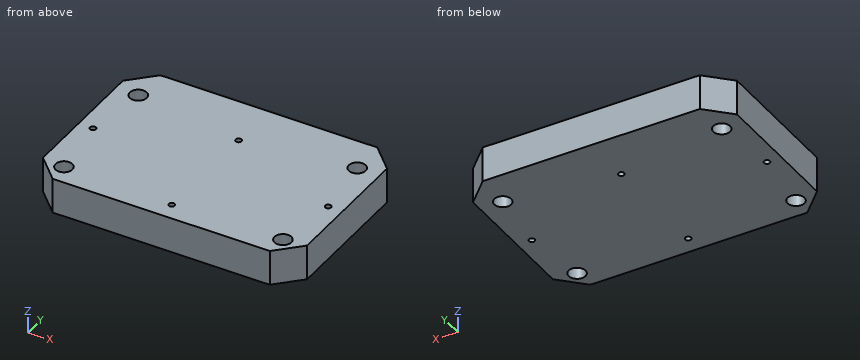
from build123d import *

# Parameters (mm, degrees)
SKETCH1_W                        = 142.628975504
SKETCH1_H                        = 98.843650928
BOSS_EXTRUDE1_DEPTH              = 19.05
CHAMFER1_SIZE                    = 12.7
F_23_64_0_35938_DIAMETER_HOLE1_D = 9.128252
HOLE1_D                          = 3.175
HOLE1_DEPTH                      = 44.45
HOLE1_CSINK_D                    = 10.16
HOLE1_CSINK_ANGLE                = 82
HOLE1_TIP                        = 0.953866233


with BuildPart() as part:
    # Sketch1 → Boss-Extrude1 (new body)
    with BuildSketch(Plane.XY):
        with Locations((0, 439.814227158)):
            Rectangle(SKETCH1_W, SKETCH1_H)
    extrude(amount=BOSS_EXTRUDE1_DEPTH)

    # Chamfer1
    chamfer1_edges = [part.edges().sort_by_distance(p)[0] for p in [
        (71.314487752, 390.392401694, 9.525),
        (-71.314487752, 390.392401694, 9.525),
        (-71.314487752, 489.236052622, 9.525),
        (71.314487752, 489.236052622, 9.525),
    ]]
    chamfer(chamfer1_edges, length=CHAMFER1_SIZE)

    # 23/64 (0.35938) Diameter Hole1 (through all)
    with Locations(Plane.XY.offset(19.05)):
        with Locations((-59.12, 469.942526688), (59.12, 469.942526688), (59.12, 401.616526688), (-59.12, 401.616526688)):
            Hole(F_23_64_0_35938_DIAMETER_HOLE1_D / 2)

    # Hole1
    with Locations(Plane(origin=(0, 0, -19.05), x_dir=(-1, 0, 0), z_dir=(0, 0, -1))):
        with Locations((63.5, 435.779526688), (-63.5, 435.779526688), (0, 461.558384256), (0, 400.075074406)):
            CounterSinkHole(HOLE1_D / 2, HOLE1_CSINK_D / 2, depth=HOLE1_DEPTH, counter_sink_angle=HOLE1_CSINK_ANGLE)
            with Locations((0, 0, -(HOLE1_DEPTH + HOLE1_TIP / 2))):  # 118° drill point
                Cone(0, HOLE1_D / 2, HOLE1_TIP, mode=Mode.SUBTRACT)


solid = part.part
Geometry: final body of the model. Coordinates: model frame, mm. Give positions to 0.01 mm unless a question says otherwise; leave off trailing zeros. Write each loop counter-clockwise with the first axis right and the second up, starting at its lowest first coordinate (ties: lowest second). Pieces come first, ordered by that corner, then holes. Notation, with made-up numbers: (70, 68.25) -> (125, 68.25) arc R16 ccw to (125, 87.25) -> close; hole circle Ø4 at (53.25, 46). An arc over 180 degrees is marked (long way). Answer as a JSON object with one key per item and string values.
1. Cut plane A-A on x = 0. Output: boundary loops of the cut face in (y, z), and give its area (3 significant figures).
Ans:
{"outline": "(390.39, 0) -> (398.49, 0) -> (398.49, 19.05) -> (390.39, 19.05) -> close; (401.66, 0) -> (459.97, 0) -> (459.97, 19.05) -> (401.66, 19.05) -> close; (463.15, 0) -> (489.24, 0) -> (489.24, 19.05) -> (463.15, 19.05) -> close", "area": "1,760 mm^2"}
2. Ray query, probe 1 along Y at (x, z) = (0, 8.75); probe 2 along X at (y, z) = (436, 5.25); probe 3 along Y at (x, z) = (-62.5, 3.75). Return the intervals inside material, ascending. Write a range as from..to.
Ans:
{"probe 1": "y = 390.39..398.49, 401.66..459.97, 463.15..489.24", "probe 2": "x = -71.31..-65.07, -61.93..61.93, 65.07..71.31", "probe 3": "y = 394.28..398.55, 404.68..434.55, 437.01..466.88, 473.01..485.35"}
3. Cut plane B-B on z = 14. Count the separate pieces of the cut face and the enclosed holes in it, and give its area (3 significant figures).
Ans:
{"separate pieces": "1", "enclosed holes": "8", "area": "13,500 mm^2"}
